Autodesk Inventor part; units mm, degrees
ref_plane "YZ Plane" through (0, 0, 0) normal (1, 0, 0) x (0, 1, 0)
ref_plane "XZ Plane" through (0, 0, 0) normal (0, 1, 0) x (-1, 0, 0)
ref_plane "XY Plane" through (0, 0, 0) normal (0, 0, 1) x (1, 0, 0)
sketch "Sketch1" plane through (0, 0, 0) normal (0, 1, 0) x (-1, 0, 0)
  line L0 (-92.5, -223.3148) -> (-223.3148, -92.5)
  line L1 (-223.3148, -92.5) -> (-223.3148, 92.5)
  line L2 (-223.3148, 92.5) -> (-92.5, 223.3148)
  line L3 (-92.5, 223.3148) -> (92.5, 223.3148)
  line L4 (92.5, 223.3148) -> (223.3148, 92.5)
  line L5 (223.3148, 92.5) -> (223.3148, -92.5)
  line L6 (223.3148, -92.5) -> (92.5, -223.3148)
  line L7 (92.5, -223.3148) -> (-92.5, -223.3148)
  circle A0 centre (0, 0) radius 46
  circle A1 centre (0, 0) radius 174
  dimension "d0" = 185
  dimension "d1" = 128
  dimension "d2" = 92
extrude "Extrusion1" add sketch "Sketch1" along normal blind 5
sketch "Sketch4" plane through (0, 5, 0) normal (0, 1, 0) x (1, 0, 0)
  circle A0 centre (0, 0) radius 174
  line L0 (0, 174) -> (0, 223.3148)
  line L1 (92.5, 223.3148) -> (-92.5, 223.3148)
  circle A1 centre (0, 198.6574) radius 12.5
  dimension "d10" = 25
extrude "Extrusion4" cut sketch "Sketch4" against normal blind 5 contours A1 L0 | L0 A1
pattern_circular "Circular Pattern1" count 4 over 360 about axis through (0, -10, 0) along (0, 1, 0) of "Extrusion4"
sketch "Sketch5" plane through (0, 5, 0) normal (0, 1, 0) x (1, 0, 0)
  line L0 (-223.3148, -92.5) -> (-92.5, -223.3148)
  line L1 (-92.5, -223.3148) -> (-66.5869, -160.755)
  circle A0 centre (0, 0) radius 174
  circle A1 centre (-79.5435, -192.0349) radius 15
  line L2 (-92.5, -223.3148) -> (92.5, -223.3148)
  circle A2 centre (0, -198.6574) radius 12.5
  line L3 (0, -211.1574) -> (0, -186.1574)
  line L4 (-44.7395, -223.3148) -> (-34.1805, -170.6098)
  line L5 (92.5, -223.3148) -> (223.3148, -92.5)
  line L6 (92.5, -223.3148) -> (66.5869, -160.755)
  circle A3 centre (79.5435, -192.0349) radius 15
  arc A4 (-79.5435, -192.0349) -> (79.5435, -192.0349) centre (0, 282.3572) ccw
  circle A5 centre (-39.4746, -197.0349) radius 10
  circle A6 centre (39.4746, -197.0349) radius 10
  line L7 (-79.5435, -207.0349) -> (-39.4746, -207.0349)
  line L8 (-79.5435, -192.0349) -> (-39.4746, -197.0349)
  line L9 (-75.8573, -177.4949) -> (-37.0171, -187.3415)
  dimension "d16" = 30
  dimension "d18" = 20
  dimension "d17" = 30
extrude "Extrusion5" cut sketch "Sketch5" against normal blind 5 contours A1 L1 | L1 A4 A1 | L8 A1 A4 | L1 A1 L8 | L9 L1 A1 | A1 A4 A5 L4 L7 | L4 A5 L7 | L1 L9 L4 A5 L8 A1 | A1 L8 A5 A4 | A5 A4 L4 | L4 A4 A5 | A5 L8 A4 | A5 L4 L8 | L9 A5 L4 | L4 A5 A4
mirror "Mirror1" about plane through (0, 0, 0) normal (1, 0, 0) of "Extrusion5"
pattern_circular "Circular Pattern2" count 4 over 360 about axis through (0, -10, 0) along (0, 1, 0) of "Extrusion5", "Mirror1"
sketch "Sketch6" plane through (0, 5, 0) normal (0, 1, 0) x (1, 0, 0)
  arc A0 (177.4949, -75.8573) -> (207.0349, -79.5435) centre (192.0349, -79.5435) ccw
  line L0 (207.0349, -79.5435) -> (207.0349, -39.4746)
  line L1 (207.0349, -79.5435) -> (177.0349, -79.5435)
  arc A1 (79.5435, -207.0349) -> (75.8573, -177.4949) centre (79.5435, -192.0349) ccw
  line L2 (75.8573, -177.4949) -> (79.5435, -192.0349)
  line L3 (0, 0) -> (79.5435, -79.5435)
  line L4 (92.5, -223.3148) -> (223.3148, -92.5)
  line L5 (92.5, -223.3148) -> (223.3148, -92.5)
  line L6 (79.5435, -79.5435) -> (157.9074, -157.9074)
  circle A2 centre (0, 0) radius 174
  line L7 (123.0366, -123.0366) -> (157.9074, -157.9074)
  arc A3 (79.5435, -192.0349) -> (140.472, -140.472) centre (-199.6567, 199.6567) ccw
  arc A4 (140.472, -140.472) -> (192.0349, -79.5435) centre (-199.6567, 199.6567) ccw
  circle A5 centre (167.5194, -111.0791) radius 5
  dimension "d26" = 10
  dimension "d27" = 481.0145
extrude "Extrusion6" cut sketch "Sketch6" against normal blind 5 contours A5 A4 | A4 A5
mirror "Mirror2" about plane through (0, 0, 0) normal (0, 0, 1) of "Extrusion6"
pattern_circular "Circular Pattern3" count 4 over 360 about axis through (0, -10, 0) along (0, 1, 0) of "Extrusion6", "Mirror2"
sketch "Sketch7" plane through (0, 5, 0) normal (0, 1, 0) x (1, 0, 0)
  arc A0 (207.0349, 79.5435) -> (177.4949, 75.8573) centre (192.0349, 79.5435) ccw
  circle A1 centre (198.6574, 0) radius 12.5
  line L0 (186.1574, 0) -> (198.6574, 0)
  arc A2 (187.3415, 37.0171) -> (207.0349, 39.4746) centre (197.0349, 39.4746) ccw
  line L1 (187.3415, 37.0171) -> (197.0349, 39.4746)
  line L2 (198.6574, 0) -> (197.0349, 39.4746)
  point P0 (0, 0)
  dimension "d33" = 39.4746
sketch "Sketch11" plane through (0, 5, 0) normal (0, 1, 0) x (1, 0, 0)
  circle A0 centre (0, 0) radius 50
  dimension "d44" = 100
extrude "Extrusion10" cut sketch "Sketch11" against normal blind 10
properties part number "Telescope_Base"
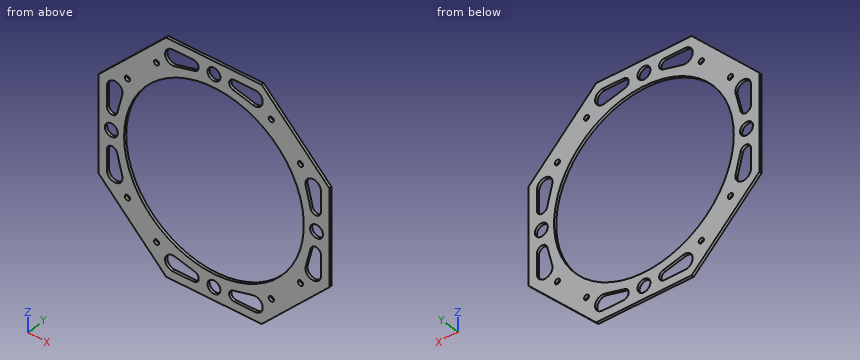
Here's how the part is built. I have some questions about the finished solid (model axes, mm). Coordinates: 2 decimals unless noted, no trailing zeros. Order: outer loops, then holes, each group sorted by start corner. A loop starts at its lowest first (then second) coordinate and runs counter-clockwise, first axis right, second up.
Item 1: For P1, Ø24, axis at x = 192.03, z = 79.54, coming from the +Y side (3 decimals); P2, Ø3, axis at x = -167.5, y = 3.5, coming from the +Z side, each with a flat end and sliding along its axis, tell me the tip position at first contact or that it passes through.
Result sheet:
P1: passes through
P2: stops at z = 149.81
Item 2: If we section it at D-D on y = 2.7: State how many separate pieces and enclosed holes the cut face has, plus the area to 3 significant figures.
Result sheet:
separate pieces: 1
enclosed holes: 21
area: 55,300 mm2
Item 3: I need wall thicknesses on line 1 (X direction, y = 0.95, z = -31.5); line 2 (Z direction, x = 113, y = 2.6); line 3 (X direction, y = 3.2, z = 114). Which ranges of each line are inside material? Lowest first, please.
Result sheet:
line 1: x = -223.31 to -203.07, -191 to -171.12, 171.12 to 191, 203.07 to 223.31
line 2: z = -202.81 to -172.14, -162.9 to -132.31, 132.31 to 162.9, 172.14 to 202.81
line 3: x = -201.81 to -171.58, -163.46 to -131.45, 131.45 to 163.46, 171.58 to 201.81
Item 4: If we section it at C-C on z = -129: List the corners of the cut face in (x, y) for me, plus the area to 3 significant figures.
Result sheet:
outline: (-186.81, 0) - (-116.77, 0) - (-116.77, 5) - (-186.81, 5) - close; (116.77, 0) - (186.81, 0) - (186.81, 5) - (116.77, 5) - close
area: 700 mm2
Item 5: If we section it at A-A on z = 0: List the corners of the cut face in (x, y) for me.
Result sheet:
outline: (-223.31, 0) - (-211.16, 0) - (-211.16, 5) - (-223.31, 5) - close; (-186.16, 0) - (-174, 0) - (-174, 5) - (-186.16, 5) - close; (174, 0) - (186.16, 0) - (186.16, 5) - (174, 5) - close; (211.16, 0) - (223.31, 0) - (223.31, 5) - (211.16, 5) - close
Item 6: If we section it at B-B on x = 0: List the corners of the cut face in (y, z) for me.
Result sheet:
outline: (0, -223.31) - (5, -223.31) - (5, -211.16) - (0, -211.16) - close; (0, -186.16) - (5, -186.16) - (5, -174) - (0, -174) - close; (0, 174) - (5, 174) - (5, 186.16) - (0, 186.16) - close; (0, 211.16) - (5, 211.16) - (5, 223.31) - (0, 223.31) - close
